CAD build for the part. Positions are in the model's coordinates, mm. A direction names the side the tool comes from. Round coordinates to 2 decimals unless told otherwise and drop trailing zeros. Loops run counter-clockwise (first coordinate to the right, second up) from the corner with the lowest first, then second, coordinate; pieces in that order, holes last.
from build123d import *

# Parameters (mm, degrees)
ESQUISSE1_W             = 270
ESQUISSE1_H             = 200
BOSS_EXTRU_1_DEPTH      = 6
ESQUISSE2_R             = 7.5
ENL_V_MAT_EXTRU_1_DEPTH = 10
ESQUISSE4_W             = 40
ESQUISSE4_H             = 6
ESQUISSE4_W_2           = 6
ESQUISSE4_H_2           = 50
ESQUISSE4_H_3           = 40
ENL_V_MAT_EXTRU_2_DEPTH = 6
ESQUISSE5_W             = 6
ESQUISSE5_H             = 25
ENL_V_MAT_EXTRU_3_DEPTH = 10
ESQUISSE6_W             = 30.179320299
ESQUISSE6_H             = 200.522044325
ENL_V_MAT_EXTRU_4_DEPTH = 169.110082981
ESQUISSE7_R             = 2.995
ENL_V_MAT_EXTRU_5_DEPTH = 3
ESQUISSE8_R             = 1.5
ENL_V_MAT_EXTRU_6_DEPTH = 13
ESQUISSE9_W             = 6
ESQUISSE9_H             = 28.5
ESQUISSE9_H_2           = 28
ESQUISSE9_H_3           = 31.5
ENL_V_MAT_EXTRU_7_DEPTH = 10


with BuildPart() as part:
    # Esquisse1 → Boss.-Extru.1 (new body)
    with BuildSketch(Plane.XY):
        Rectangle(ESQUISSE1_W, ESQUISSE1_H)
    extrude(amount=BOSS_EXTRU_1_DEPTH)

    # Esquisse2 → Enlèv. mat.-Extru.1 (cut)
    with BuildSketch(Plane(origin=(0, 0, 0), x_dir=(-1, 0, 0), z_dir=(0, 0, -1))):
        with Locations((110, -75)):
            Circle(ESQUISSE2_R)
    extrude(amount=-ENL_V_MAT_EXTRU_1_DEPTH, mode=Mode.SUBTRACT)

    # Esquisse4 → Enlèv. mat.-Extru.2 (cut)
    with BuildSketch(Plane.XY.offset(6)):
        with Locations((-75, -97)):
            Rectangle(ESQUISSE4_W, ESQUISSE4_H)
        with Locations((5, -97)):
            Rectangle(ESQUISSE4_W, ESQUISSE4_H)
        with Locations((85, -97)):
            Rectangle(ESQUISSE4_W, ESQUISSE4_H)
        with Locations((-75, 97)):
            Rectangle(ESQUISSE4_W, ESQUISSE4_H)
        with Locations((5, 97)):
            Rectangle(ESQUISSE4_W, ESQUISSE4_H)
        with Locations((85, 97)):
            Rectangle(ESQUISSE4_W, ESQUISSE4_H)
        with Locations((132, -75)):
            Rectangle(ESQUISSE4_W_2, ESQUISSE4_H_2)
        with Locations((132, 75)):
            Rectangle(ESQUISSE4_W_2, ESQUISSE4_H_2)
        with Locations((132, 0)):
            Rectangle(ESQUISSE4_W_2, ESQUISSE4_H_3)
    extrude(amount=-ENL_V_MAT_EXTRU_2_DEPTH, mode=Mode.SUBTRACT)

    # Esquisse5 → Enlèv. mat.-Extru.3 (cut)
    with BuildSketch(Plane(origin=(0, 0, 0), x_dir=(-1, 0, 0), z_dir=(0, 0, -1))):
        with Locations((72, -55)):
            Rectangle(ESQUISSE5_W, ESQUISSE5_H)
        with Locations((72, 0)):
            Rectangle(ESQUISSE5_W, ESQUISSE5_H)
        with Locations((72, 55)):
            Rectangle(ESQUISSE5_W, ESQUISSE5_H)
    extrude(amount=-ENL_V_MAT_EXTRU_3_DEPTH, mode=Mode.SUBTRACT)

    # Esquisse6 → Enlèv. mat.-Extru.4 (cut, through all)
    with BuildSketch(Plane.XY.offset(6)):
        with Locations((120.08966015, -0.261022163)):
            Rectangle(ESQUISSE6_W, ESQUISSE6_H)
    extrude(amount=-ENL_V_MAT_EXTRU_4_DEPTH, mode=Mode.SUBTRACT)

    # Esquisse7 → Enlèv. mat.-Extru.5 (cut)
    with BuildSketch(Plane(origin=(0, 0, 0), x_dir=(-1, 0, 0), z_dir=(0, 0, -1))):
        with Locations((-45, 97)):
            Circle(ESQUISSE7_R)
        with Locations((35, 97)):
            Circle(ESQUISSE7_R)
        with Locations((115, 97)):
            Circle(ESQUISSE7_R)
        with Locations((-45, -97)):
            Circle(ESQUISSE7_R)
        with Locations((35, -97)):
            Circle(ESQUISSE7_R)
        with Locations((115, -97)):
            Circle(ESQUISSE7_R)
    extrude(amount=-ENL_V_MAT_EXTRU_5_DEPTH, mode=Mode.SUBTRACT)

    # Esquisse8 → Enlèv. mat.-Extru.6 (cut)
    with BuildSketch(Plane(origin=(0, 0, 0), x_dir=(-1, 0, 0), z_dir=(0, 0, -1))):
        with Locations((-45, 97)):
            Circle(ESQUISSE8_R)
        with Locations((35, 97)):
            Circle(ESQUISSE8_R)
        with Locations((115, 97)):
            Circle(ESQUISSE8_R)
        with Locations((-45, -97)):
            Circle(ESQUISSE8_R)
        with Locations((35, -97)):
            Circle(ESQUISSE8_R)
        with Locations((115, -97)):
            Circle(ESQUISSE8_R)
    extrude(amount=-ENL_V_MAT_EXTRU_6_DEPTH, mode=Mode.SUBTRACT)

    # Esquisse9 → Enlèv. mat.-Extru.7 (cut)
    with BuildSketch(Plane(origin=(0, 0, 0), x_dir=(-1, 0, 0), z_dir=(0, 0, -1))):
        with Locations((132, -79.75)):
            Rectangle(ESQUISSE9_W, ESQUISSE9_H)
        with Locations((132, -26.5)):
            Rectangle(ESQUISSE9_W, ESQUISSE9_H_2)
        with Locations((132, 31.25)):
            Rectangle(ESQUISSE9_W, ESQUISSE9_H_3)
    extrude(amount=-ENL_V_MAT_EXTRU_7_DEPTH, mode=Mode.SUBTRACT)


solid = part.part
Item 1: Cut at A-A (x = -72). List the corners of the cut face in (y, z).
Verdict:
outline: (-94, 0) - (-67.5, 0) - (-67.5, 6) - (-94, 6) - close; (-42.5, 0) - (-12.5, 0) - (-12.5, 6) - (-42.5, 6) - close; (12.5, 0) - (42.5, 0) - (42.5, 6) - (12.5, 6) - close; (67.5, 0) - (94, 0) - (94, 6) - (67.5, 6) - close
Item 2: Wall check: L1, parallel to X at y = -97, z = 5.3; L2, parallel to Y at x = 45, z = 4.55; L3, parallel to X at y = -22.5, z = 5.35. Give the ranges that are in metal, low to high.
Verdict:
L1: x = -135 to -116.5, -113.5 to -95, -55 to -36.5, -33.5 to -15, 25 to 43.5, 46.5 to 65
L2: y = -100 to -98.5, -95.5 to 95.5, 98.5 to 100
L3: x = -129 to 105
Item 3: Cut at D-D (z = 3.95). State how many separate pieces and enclosed holes the cut face has, plus the area to 3 significant figures.
Verdict:
separate pieces: 1
enclosed holes: 10
area: 45,400 mm2
Item 4: Flat gauge pins, fed straight in: P1, Ø1.8, axis at y = -96, z = 2, coming from the +X side; P2, Ø5, axis at x = -115, y = -97, coming from the -Z side; P3, Ø1.8, axis at x = 3.5, z = 4.5, coming from the -Y side. Where does each tip first touch, or does it go through?
Verdict:
P1: stops at x = 65
P2: stops at z = 3
P3: stops at y = -94
Item 5: 3-axis set-ups, long thin cutter, end or side, ignore diameter. For faces 1 (the flat face through (-36.3, -98.3, 3)), 2 (the flat face through (-75, -94, 3)), 3 (the flat face through (-132, -94, 3)): which of +Z, -Z, +X, -X, +Y, -Y reach the whole face in a straight line?
Verdict:
face 1: -Z
face 2: +Z, -Z, -Y
face 3: +Z, -Z, -X
Item 6: Cut at B-B (y = -45). List the corners of the cut face in (x, z).
Verdict:
outline: (-135, 0) - (-75, 0) - (-75, 6) - (-135, 6) - close; (-69, 0) - (105, 0) - (105, 6) - (-69, 6) - close
Item 7: Cut at C-C (y = -75). List the corners of the cut face in (x, z), plus the area to 3 significant figures.
Verdict:
outline: (-129, 0) - (-117.5, 0) - (-117.5, 6) - (-129, 6) - close; (-102.5, 0) - (105, 0) - (105, 6) - (-102.5, 6) - close
area: 1,310 mm2
Item 8: Mould opens along X. For faces 4 (the flat face through (-132, -40.5, 3)), 5 (the flat face through (-55, 97, 3)), 6 (the flat face through (43.7, -98.3, 3)) say: released by +X, released by -X, zero draft, split by the parting line, or undercut.
Verdict:
face 4: zero draft
face 5: undercut
face 6: undercut
